Here's the drawing with two shaded views (mm, measured from the low corner). I have some questions. Give positions to 0.01 mm unless a question says otherwise; leave off trailing zeros. Write each loop counter-clockwise with the first axis right and the second up, starting at its lowest first coordinate (ties: lowest second). Pieces come first, ordered by that corner, then holes. Notation, with made-up numbers: (23.5, -20.5) -> (52.5, -20.5) arc R23 ccw to (52.5, 1.5) -> close; hole circle Ø9 at (-21, 85.5). An arc over 180 degrees is marked (long way). One line per item, written item: value.
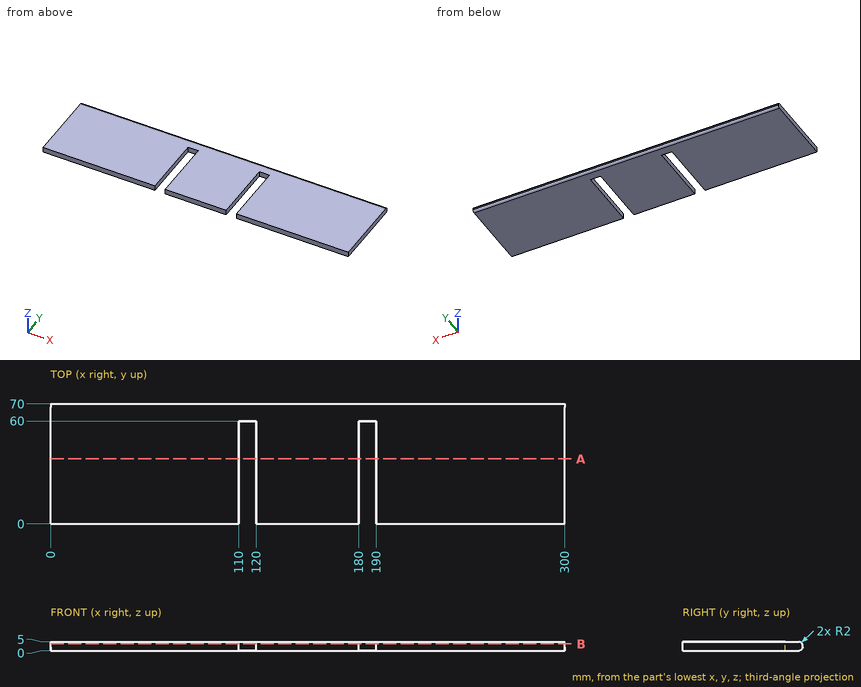
1) If we section it at B-B (z = 3.9): Write out the boundary of the cut face in (x, y), and give its area (3 significant figures).
Answer list:
outline: (0, 0) -> (110, 0) -> (110, 60) -> (120, 60) -> (120, 0) -> (180, 0) -> (180, 60) -> (190, 60) -> (190, 0) -> (300, 0) -> (300, 69.79) -> (0, 69.79) -> close
area: 19,700 mm^2
2) I need wall thicknesses on L1, parallel to X at y = 54, z = 3.1; L2, parallel to Y at x = 143.5, z = 3.1; L3, parallel to Y at x = 217, z = 0.4. Which ranges of each line are inside material? Lowest first, please.
Answer list:
L1: x = 0 to 110, 120 to 180, 190 to 300
L2: y = 0 to 70
L3: y = 0 to 69.2
3) If we section it at A-A (y = 38): Write out the boundary of the cut face in (x, z), and give its area (3 significant figures).
Answer list:
outline: (0, 0) -> (110, 0) -> (110, 5) -> (0, 5) -> close; (120, 0) -> (180, 0) -> (180, 5) -> (120, 5) -> close; (190, 0) -> (300, 0) -> (300, 5) -> (190, 5) -> close
area: 1,400 mm^2
4) Will these pins go through, and if not, where does the flat tip stop? pin 1 (2.5 mm diameter, centred on x = 116.5, z = 2.5, fed in from -Y); pin 2 (1.5 mm diameter, centred on x = 182.5, y = 9.5, fed in from -Z).
Answer list:
pin 1: stops at y = 60
pin 2: passes through
